```python
from build123d import *

# Parameters (mm, degrees)
F2_DEPTH = 5
F3_R     = 1.5
F4_R     = 4.99999
F6_D     = 3.25


# Not quite as in the source:
# - a fillet or chamfer is up to 0.001 mm smaller than in the source, because OpenCascade refuses the exact size


with BuildPart() as f2:
    # F1 (on Right) → F2 (new body, symmetric)
    with BuildSketch(Plane.YZ):
        with BuildLine():
            Line((-4.5, 12.592475), (-7.7353845436, 12.592475))
            ThreePointArc((-7.7353845436, 12.592475), (-7.9922437092, 12.4953707173), (-8.099967, 12.242781))
            Line((-8.099967, 12.242781), (-8.099967, 10.260188))
            ThreePointArc((-8.099967, 10.260188), (-8.0733249886, 10.126249564), (-7.9974549592, 10.0127020408))
            Line((-7.9974549828, 10.0127020172), (-4.0719369828, 6.0871840172))
            ThreePointArc((-4.0719369592, 6.0871840408), (-3.958389436, 6.0113140114), (-3.824451, 5.984672))
            Line((-3.824451, 5.984672), (-0.949996, 5.984672))
            Line((-0.949996, 5.984672), (0.949996, 5.984672))
            Line((0.949996, 5.984672), (3.824451, 5.984672))
            ThreePointArc((3.824451, 5.984672), (3.958389436, 6.0113140114), (4.0719369592, 6.0871840408))
            Line((4.0719369828, 6.0871840172), (7.9974549828, 10.0127020172))
            ThreePointArc((7.9974549592, 10.0127020408), (8.0733249886, 10.126249564), (8.099967, 10.260188))
            Line((8.099967, 10.260188), (8.099967, 12.242781))
            ThreePointArc((8.099967, 12.242781), (7.9922437092, 12.4953707173), (7.7353845436, 12.592475))
            Line((7.7353845436, 12.592475), (4.5, 12.592475))
            Line((4.5, 12.592475), (-1, 12.592475))
            Line((-1, 12.592475), (-1, 22.99994))
            Line((-1, 22.99994), (-3, 22.99994))
            Line((-3, 22.99994), (-3, 12.592475))
            Line((-3, 12.592475), (-4.5, 12.592475))
        make_face()
    extrude(amount=F2_DEPTH, both=True)

    # F3
    f3_edges = [f2.edges().sort_by_distance(p)[0] for p in [
        (0, -3, 12.592475),
        (0, -1, 12.592475),
    ]]
    fillet(f3_edges, radius=F3_R)

    # F4 (radius 5 in the source; OpenCascade refuses exactly that, so slightly less here)
    f4_edges = [f2.edges().sort_by_distance(p)[0] for p in [
        (5, -2, 22.99994),
        (-5, -2, 22.99994),
    ]]
    fillet(f4_edges, radius=F4_R)

    # F6 (through all)
    with Locations(Plane(origin=(0, -1, 0), x_dir=(-1, 0, 0), z_dir=(0, 1, 0))):
        with Locations((0, 18.99994)):
            Hole(F6_D / 2)


solid = f2.part
```
Could you check a few things on this model? Use its own coordinates, in mm. A direction names the side the tool comes from. Give positions to 0.01 mm unless a question says otherwise; leave off trailing zeros. Write each loop counter-clockwise with the first axis right and the second up, starting at its lowest first coordinate (ties: lowest second). Pieces come first, ordered by that corner, then holes. Notation, with made-up numbers: (47, 17) - (102, 17) arc R23 ccw to (102, 46) - close; hole circle Ø11 at (58.25, 8). An arc over 180 degrees is marked (long way). One line per item, written item: value. Start each with the question number.
Item 1: Imagine slicing it at D-D, the plane z = 15.25. List the corners of the cut face in (x, y) for me.
Item 2: Imagine slicing it at C-C, the plane y = 3.25. List the corners of the cut face in (x, z) for me, and give its area (3 significant figures).
Item 3: I'm going to push flat-ended pins straight in: pin 1 (1.5 mm diameter, centred on x = 4, y = 4, fed in from +Z); pin 2 (5 mm diameter, centred on x = 0, z = 19, fed in from -Y); pin 3 (1.5 mm diameter, centred on x = 1, y = -4.5, fed in from +Z). Where does each tip first touch, or does it pass through?
Item 4: Please list where these lines run through material, in increasing order: line 1 (Z direction, x = 0, y = -1.7); line 2 (Z direction, x = 3.5, y = 3.25); line 3 (Y direction, x = 1.5, z = 19.75). Write a range as from..to.
Item 5: Imagine slicing it at A-A, the plane x = -1.25. List the corners of the cut face in (y, z) for me.
Item 6: Imagine slicing it at B-B, the plane z = 19.25. List the corners of the cut face in (x, y) for me, and give its area (3 significant figures).
Item 7: Which directions (+Z, -Z, +X, -X, +Y, -Y) give clear straight access to the entire face, cutting with the end or side of a thin tool? Please do faces 5 (the face through (0, -6, 12.592)), 6 (the face through (0.07, 6.007, 8.022)), 7 (the face through (1, -1, 17)).
Item 8: If we mould it in two halves opening along Z, with no side actions, what happens to faces 1 (the face through (1.2, -3, 17.6)), 2 (the face through (0, 4, 12.592)), 3 (the face through (0.07, -6.062, 8.077)), 4 (the face through (-0.21, -2.01, 20.61))? For each: +Z half, -Z half, draft (parallel to the pull), parting line (faces both ways), or undercut.
Geometry says:
1. outline: (-5, -3) - (5, -3) - (5, -1) - (-5, -1) - close
2. outline: (-5, 5.98) - (5, 5.98) - (5, 12.59) - (-5, 12.59) - close
2. area: 66.1 mm^2
3. pin 1: z = 12.59
3. pin 2: y = -3
3. pin 3: z = 12.79
4. line 1: 5.98..17.37, 20.62..23
4. line 2: 5.98..12.59
4. line 3: -3..-1
5. outline: (-8.1, 10.26) arc R0.35 ccw to (-8, 10.01) - (-4.07, 6.09) arc R0.35 ccw to (-3.82, 5.98) - (3.82, 5.98) arc R0.35 ccw to (4.07, 6.09) - (8, 10.01) arc R0.35 ccw to (8.1, 10.26) - (8.1, 12.24) arc R0.35 ccw to (7.74, 12.59) - (0.5, 12.59) arc R1.5 cw to (-1, 14.09) - (-1, 17.96) - (-3, 17.96) - (-3, 14.09) arc R1.5 cw to (-4.5, 12.59) - (-7.74, 12.59) arc R0.35 ccw to (-8.1, 12.24) - close; (-3, 20.04) - (-1, 20.04) - (-1, 22.84) - (-3, 22.84) - close
6. outline: (-4.84, -3) - (-1.61, -3) - (-1.61, -1) - (-4.84, -1) - close; (1.61, -3) - (4.84, -3) - (4.84, -1) - (1.61, -1) - close
6. area: 12.9 mm^2
7. face 5: +Z, +X, -X, -Y
7. face 6: -Z, +X, -X, +Y
7. face 7: +Z, +X, -X, +Y
8. face 1: draft
8. face 2: +Z half
8. face 3: -Z half
8. face 4: undercut
